```python
from build123d import *

# Parameters (mm, degrees)
F0_W     = 12
F0_H     = 30
F0_W_2   = 8
F0_H_2   = 3
F1_DEPTH = 3
F2_R     = 1


with BuildPart() as f1:
    # F0 (on Right) → F1 (new body)
    with BuildSketch(Plane.YZ):
        Polygon((14, -37), (14, 37), (6, 37), (-6, 37), (-14, 37), (-14, -37), (-6, -37), (6, -37), align=None)
        with BuildLine():
            Line((-10.1, -6.8), (-10.1, 3.2))
            ThreePointArc((-10.1, 3.2), (-8.7, 4.6), (-7.3, 3.2))
            Line((-7.3, 3.2), (-7.3, -6.8))
            ThreePointArc((-7.3, -6.8), (-8.7, -8.2), (-10.1, -6.8))
        make_face(mode=Mode.SUBTRACT)
        with BuildLine():
            ThreePointArc((-5, -17), (0, -12), (5, -17))
            Line((5, -17), (5, -27))
            ThreePointArc((5, -27), (0, -32), (-5, -27))
            Line((-5, -27), (-5, -17))
        make_face(mode=Mode.SUBTRACT)
        with BuildLine():
            ThreePointArc((7.3, 3.2), (8.7, 4.6), (10.1, 3.2))
            Line((10.1, 3.2), (10.1, -6.8))
            ThreePointArc((10.1, -6.8), (8.7, -8.2), (7.3, -6.8))
            Line((7.3, -6.8), (7.3, 3.2))
        make_face(mode=Mode.SUBTRACT)
        with Locations((0, 18)):
            Rectangle(F0_W, F0_H, mode=Mode.SUBTRACT)
        with Locations((10, 38.5)):
            Rectangle(F0_W_2, F0_H_2)
        with Locations((10, -38.5)):
            Rectangle(F0_W_2, F0_H_2)
        with Locations((-10, 38.5)):
            Rectangle(F0_W_2, F0_H_2)
        with Locations((-10, -38.5)):
            Rectangle(F0_W_2, F0_H_2)
    extrude(amount=F1_DEPTH)

    # F2
    f2_edges = [f1.edges().sort_by_distance(p)[0] for p in [
        (1.5, 6, 33),
        (1.5, -6, 33),
        (1.5, -6, 3),
        (1.5, 6, 3),
    ]]
    fillet(f2_edges, radius=F2_R)


solid = f1.part
```
Check sheet for the modelled part. Datum: model origin and axes. Units: mm. A direction names the side the tool comes from. Give positions to 0.01 mm unless a question says otherwise; leave off trailing zeros. Write each loop counter-clockwise with the first axis right and the second up, starting at its lowest first coordinate (ties: lowest second). Pieces come first, ordered by that corner, then holes.
Item 1: Cross-section at A-A (y = 0). Enter the section's corners in (x, z), and give its area (3 significant figures).
Item 2: Draft check along Z on faces 5 (the face through (1.5, 8.7, 4.6)), 6 (the face through (1, 0, -37)), 7 (the face through (0, 0, 1)), 8 (the face through (1, 0, 33)). Enter one of: released by +Z, released by -Z, zero draft, split by the parting line, or undercut.
Item 3: Cross-section at D-D (x = 1). Count the separate pieces of the cut face and the enclosed holes in it, and give its area (3 significant figures).
Item 4: Cross-section at B-B (z = 22). Enter the section's corners in (x, y).
Item 5: Gauge pin test, flat ends, axial feed: pin 1 (2 mm diameter, centred on y = -2, z = -3, fed in from -X); pin 2 (0.9 mm diameter, centred on x = 1.5, y = 1, fed in from +Z). Record the tip position at first contact, or that the pin passes through.
Item 6: Scan lines: L1, parallel to Y at x = 2.1, z = -7; L2, parallel to Y at x = 1.2, z = 6; L3, parallel to Z at x = 0.95, y = 1. Record each from-to range of solid material in increasing order.
Item 7: Access from +Z, -Z, +X, -X, +Y, -Y to the whole of each face (thin tool, end or side, straight path). Record for faces 1 (the face through (1, 10.1, -2)), 2 (the face through (1, 6, 38)), 3 (the face through (1, 14, -1)), 4 (the face through (1, 6, -39)).
Item 8: Cross-section at C-C (y = 8.7). Enter the section's corners in (x, z).
Report:
1. outline: (0, -37) - (3, -37) - (3, -32) - (0, -32) - close; (0, -12) - (3, -12) - (3, 3) - (0, 3) - close; (0, 33) - (3, 33) - (3, 37) - (0, 37) - close
1. area: 72.0 mm2
2. face 5: undercut
2. face 6: released by -Z
2. face 7: zero draft
2. face 8: undercut
3. separate pieces: 1
3. enclosed holes: 4
3. area: 1,560 mm2
4. outline: (0, -14) - (3, -14) - (3, -6) - (0, -6) - close; (0, 6) - (3, 6) - (3, 14) - (0, 14) - close
5. pin 1: stops at x = 0
5. pin 2: stops at z = 37
6. L1: y = -14 to -10.09, -7.31 to 7.31, 10.09 to 14
6. L2: y = -14 to -6, 6 to 14
6. L3: z = -37 to -31.9, -12.1 to 3, 33 to 37
7. face 1: +X, -X
7. face 2: +Z, +X, -X
7. face 3: +Z, -Z, +X, -X, +Y
7. face 4: -Z, +X, -X
8. outline: (0, -40) - (3, -40) - (3, -8.2) - (0, -8.2) - close; (0, 4.6) - (3, 4.6) - (3, 40) - (0, 40) - close
